Here's how the part is built. I have some questions about the finished solid (model axes, mm). A direction names the side the tool comes from. Round coordinates to 2 decimals unless told otherwise and drop trailing zeros. Order: outer loops, then holes, each group sorted by start corner. A loop starts at its lowest first (then second) coordinate and runs counter-clockwise, first axis right, second up. Notation, with made-up numbers: M -21.75,70 L 4.25,70 A24 ccw 4.25,82 Z; hole C 0.5,-11 d11. An arc over 180 degrees is marked long. Write item = value, one per line. Start each with the question number.
Item 1: I'm going to push flat-ended pins straight in: P1, Ø1.6, axis at x = -2, y = 0, coming from the -Z side; P2, Ø3.5, axis at y = -0.5, z = 0, coming from the -X side; P3, Ø1, axis at x = 11.5, y = -1, coming from the -Z side. Where does each tip first touch, or does it pass through?
Item 2: I want a section at B-B, the plane z = 0. List the corners of the cut face in (x, y) for me, plus the area to 3 significant figures.
Item 3: For faces 1 (the face through (-1.49, 0.01, 4)), 2 (the face through (-1.49, 0.01, 3.75)), 3 (the face through (-0.5, -0.6, 5.5)), 4 (the face through (-0.5, 0.6, -5.5)), which set-ups out of +Z, -Z, +X, -X, +Y, -Y let a thin tool reach every point of the face, with its end or its side?
Item 4: I want a section at C-C, the plane x = 8.25. List the corners of the cut face in (y, z) for me.
Item 5: I want a section at D-D, the plane z = -3.75. List the corners of the cut face in (x, y) for me, plus the area to 3 significant figures.
Item 6: I want a section at A-A, the plane y = 0. State how many separate pieces and enclosed holes the cut face has, plus the area to 3 significant figures.
Item 7: We'd pull the mould along Y, two halves only. Please class faces 5 (the face through (-1.49, 0.01, -4)), 6 (the face through (0, 0, 5.5)), 7 (the face through (6, -5, 0)): pulls with the +Y half, pulls with the -Y half, needs draft (parallel to the pull), parting line crosses it, or undercut.
Item 8: Please list where these lines run through material, in increasing order: L1, parallel to Y at x = -2.15, z = -4.15; L2, parallel to X at y = -0.5, z = 3.25; L3, parallel to Y at x = -1.35, z = 0.
```python
from build123d import *

# Parameters (mm, degrees)
SALIENTE_EXTRUIR1_DEPTH = 13.5
SALIENTE_EXTRUIR2_START = 1
SALIENTE_EXTRUIR2_DEPTH = 1
CROQUIS3_R              = 2.5
CROQUIS3_R_2            = 0.5
SALIENTE_EXTRUIR3_DEPTH = 1
REDONDEO1_R             = 0.25
CORTAR_EXTRUIR1_START   = -14.5
CROQUIS3_2_R            = 0.5
CORTAR_EXTRUIR1_DEPTH   = 14.5
CROQUIS4_R              = 0.5
SALIENTE_EXTRUIR4_DEPTH = 0.25
MATRIZL1_COUNT          = 2
MATRIZL1_PITCH          = 8


with BuildPart() as part:
    # Croquis1 → Saliente-Extruir1 (new body)
    with BuildSketch(Plane(origin=(0, 0, 0), x_dir=(0, 0, -1), z_dir=(1, 0, 0))):
        with BuildLine():
            Line((-3.31662479, 5), (3.31662479, 5))
            ThreePointArc((3.31662479, 5), (6, 0), (3.31662479, -5))
            Line((3.31662479, -5), (-3.31662479, -5))
            ThreePointArc((-3.31662479, -5), (-6, 0), (-3.31662479, 5))
        make_face()
    extrude(amount=SALIENTE_EXTRUIR1_DEPTH)

    # Croquis2 → Saliente-Extruir2 (add)
    with BuildSketch(Plane.ZY.offset(SALIENTE_EXTRUIR2_START)):
        with BuildLine():
            Line((-4.969924623, 0.6), (-4.969924623, -0.6))
            Line((-4.969924623, -0.6), (-5.969924623, -0.6))
            ThreePointArc((-5.969924623, -0.6), (-5.138093031, -3.098386677), (-3.31662479, -5))
            Line((-3.31662479, -5), (3.31662479, -5))
            ThreePointArc((3.31662479, -5), (5.138093031, -3.098386677), (5.969924623, -0.6))
            Line((5.969924623, -0.6), (4.969924623, -0.6))
            Line((4.969924623, -0.6), (4.969924623, 0.6))
            Line((4.969924623, 0.6), (5.969924623, 0.6))
            ThreePointArc((5.969924623, 0.6), (5.138093031, 3.098386677), (3.31662479, 5))
            Line((3.31662479, 5), (-3.31662479, 5))
            ThreePointArc((-3.31662479, 5), (-5.138093031, 3.098386677), (-5.969924623, 0.6))
            Line((-5.969924623, 0.6), (-4.969924623, 0.6))
        make_face()
    extrude(amount=-SALIENTE_EXTRUIR2_DEPTH)

    # Croquis3 → Saliente-Extruir3 (add)
    with BuildSketch(Plane.ZY.offset(1)):
        Circle(CROQUIS3_R)
        Circle(CROQUIS3_R_2, mode=Mode.SUBTRACT)
    extrude(amount=SALIENTE_EXTRUIR3_DEPTH)

    # Redondeo1
    redondeo1_edges = [part.edges().sort_by_distance(p)[0] for p in [
        (-2, 0, -2.5),
    ]]
    fillet(redondeo1_edges, radius=REDONDEO1_R)

    # Croquis3<2> → Cortar-Extruir1 (cut)
    with BuildSketch(Plane.ZY.offset(1).offset(CORTAR_EXTRUIR1_START)):
        with Locations(Location((0, 0, 0), (0, 0, 180))):
            Circle(CROQUIS3_2_R)
    extrude(amount=CORTAR_EXTRUIR1_DEPTH, mode=Mode.SUBTRACT)

    # Croquis4 → Saliente-Extruir4 (add)
    with BuildSketch(Plane.XY.offset(4)):
        Polygon((-2.55, 0.75), (-1, 0.75), (-1, -0.75), (-2.55, -0.75), (-2.8, -0.5), (-2.8, 0.5), align=None)
        with Locations((-2.15, 0)):
            Circle(CROQUIS4_R, mode=Mode.SUBTRACT)
    saliente_extruir4 = extrude(amount=-SALIENTE_EXTRUIR4_DEPTH)

    # MatrizL1: Saliente-Extruir4 ×2
    with Locations(*[(0, 0, -i * MATRIZL1_PITCH) for i in range(1, MATRIZL1_COUNT)]):
        add(saliente_extruir4)


solid = part.part
```
Filled in:
q1.P1 = -4.25
q1.P2 = -2
q1.P3 = -5.98
q2.outline = M -2,-2.25 A0.25 ccw -1.75,-2.5 L -1,-2.5 L -1,-5 L 13.5,-5 L 13.5,-0.5 L -2,-0.5 Z; M -2,0.5 L 13.5,0.5 L 13.5,5 L -1,5 L -1,2.5 L -1.75,2.5 A0.25 ccw -2,2.25 Z
q2.area = 134 mm^2
q3.face_1 = +Z, -X, +Y, -Y
q3.face_2 = -X, +Y, -Y
q3.face_3 = +Z, -X
q3.face_4 = -Z, -X
q4.outline = M -5,-3.32 A6 ccw 5,-3.32 L 5,3.32 A6 ccw -5,3.32 Z; hole C 0,0 d1
q5.outline = M -1,-4.68 L 13.5,-4.68 L 13.5,4.68 L -1,4.68 Z
q5.area = 136 mm^2
q6.separate_pieces = 4
q6.enclosed_holes = 0
q6.area = 162 mm^2
q7.face_5 = needs draft
q7.face_6 = undercut
q7.face_7 = pulls with the -Y half
q8.L1 = -0.75 to -0.5, 0.5 to 0.75
q8.L2 = -1 to 13.5
q8.L3 = -2.5 to -0.5, 0.5 to 2.5
